Verification items for the finished model (mm, model axes). Round coordinates to 2 decimals unless told otherwise and drop trailing zeros. Loops run counter-clockwise (first coordinate to the right, second up) from the corner with the lowest first, then second, coordinate; pieces in that order, holes last.
Autodesk Inventor part; units mm, degrees
ref_plane "Work Plane1" through (37.5, 25, 0) normal (0, 1, 0) x (-1, 0, 0)
ref_plane "YZ Plane" through (0, 0, 0) normal (1, 0, 0) x (0, 1, 0)
ref_plane "XZ Plane" through (0, 0, 0) normal (0, 1, 0) x (-1, 0, 0)
ref_plane "Work Plane1" through (37.5, 25, 0) normal (0, 1, 0) x (-1, 0, 0)
sketch "Sketch1" plane through (37.5, 25, 0) normal (0, 1, 0) x (-1, 0, 0)
  line L0 (0, 0) -> (75, 0)
  line L1 (75, 0) -> (75, 100)
  line L2 (0, 100) -> (75, 100)
  line L3 (0, 0) -> (0, 100)
  circle A0 centre (6.75, 86) radius 2.7
  circle A1 centre (68.25, 86) radius 2.7
  circle A2 centre (68.25, 21.25) radius 2.7
  circle A3 centre (6.75, 21.25) radius 2.7
  line L4 (3, 3) -> (3, 17.5)
  line L5 (3, 17.5) -> (10.5, 17.5)
  line L6 (10.5, 17.5) -> (10.5, 25)
  line L7 (10.5, 25) -> (3, 25)
  line L8 (3, 25) -> (3, 77.25)
  arc A4 (8, 82.25) -> (3, 77.25) centre (8, 77.25) ccw
  line L9 (8, 82.25) -> (10.5, 82.25)
  line L10 (10.5, 82.25) -> (10.5, 89.75)
  line L11 (10.5, 89.75) -> (8, 89.75)
  arc A5 (3, 94.75) -> (8, 89.75) centre (8, 94.75) ccw
  line L12 (3, 94.75) -> (3, 97)
  line L13 (3, 97) -> (72, 97)
  line L14 (72, 97) -> (72, 94.75)
  arc A6 (67, 89.75) -> (72, 94.75) centre (67, 94.75) ccw
  line L15 (67, 89.75) -> (64.5, 89.75)
  line L16 (64.5, 89.75) -> (64.5, 82.25)
  line L17 (64.5, 82.25) -> (67, 82.25)
  arc A7 (72, 77.25) -> (67, 82.25) centre (67, 77.25) ccw
  line L18 (72, 77.25) -> (72, 25)
  line L19 (72, 25) -> (64.5, 25)
  line L20 (64.5, 25) -> (64.5, 17.5)
  line L21 (64.5, 17.5) -> (72, 17.5)
  line L22 (72, 17.5) -> (72, 3)
  line L23 (72, 3) -> (3, 3)
  line L24 (72, 55) -> (3, 55)
  point P0 (37.5, 0)
  dimension "d0" = 42
extrude "Extrusion1" add sketch "Sketch1" along normal blind 3 contours L3 L2 L1 L0 | L4 L5 L6 L7 L8 L24 L18 L19 L20 L21 L22 L23
properties part number "plytka"
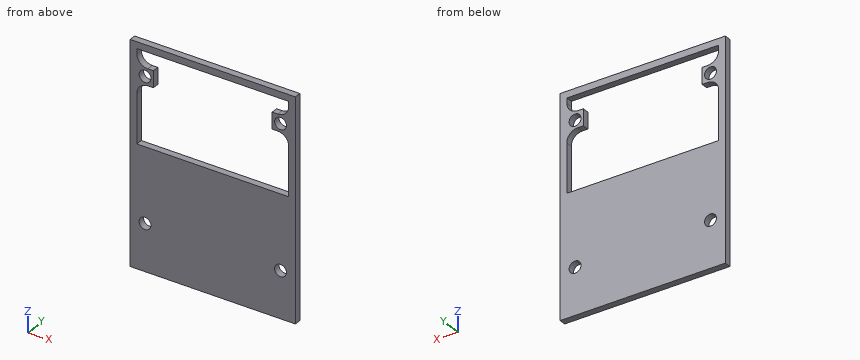
1. Section check C-C (z = 86). Enter the section's corners in (x, y).
2. Section check D-D (y = 27.45). Enter the section's corners in (x, z).
3. Section check B-B (x = 6). Enter the section's corners in (y, z), then the cut area to 3 significant figures.
4. Gauge pin test, flat end, axial feed: P1, Ø12, axis at x = -22, z = 64, coming from the -Y side. Record the tip position at first contact, or that the pin passes through.
5. Section check A-A (z = 21.25). Enter the section's corners in (x, y), then the cut area to 3 significant figures.
6. Scan lines: L1, parallel to X at y = 27, z = 67; L2, parallel to Z at x = -30.75, y = 26.1; L3, parallel to Z at x = 33.5, y = 25.6. Record each from-to range of solid material in increasing order.
Taken from the geometry:
1. outline: (-37.5, 25) - (-33.45, 25) - (-33.45, 28) - (-37.5, 28) - close; (-28.05, 25) - (-27, 25) - (-27, 28) - (-28.05, 28) - close; (27, 25) - (28.05, 25) - (28.05, 28) - (27, 28) - close; (33.45, 25) - (37.5, 25) - (37.5, 28) - (33.45, 28) - close
2. outline: (-37.5, 0) - (37.5, 0) - (37.5, 100) - (-37.5, 100) - close; hole (-34.5, 55) - (34.5, 55) - (34.5, 77.25) arc R5 ccw to (29.5, 82.25) - (27, 82.25) - (27, 89.75) - (29.5, 89.75) arc R5 ccw to (34.5, 94.75) - (34.5, 97) - (-34.5, 97) - (-34.5, 94.75) arc R5 ccw to (-29.5, 89.75) - (-27, 89.75) - (-27, 82.25) - (-29.5, 82.25) arc R5 ccw to (-34.5, 77.25) - close; hole circle Ø5.4 at (-30.75, 21.25); hole circle Ø5.4 at (-30.75, 86); hole circle Ø5.4 at (30.75, 21.25); hole circle Ø5.4 at (30.75, 86)
3. outline: (25, 0) - (28, 0) - (28, 55) - (25, 55) - close; (25, 97) - (28, 97) - (28, 100) - (25, 100) - close
3. area: 174 mm2
4. P1: passes through
5. outline: (-37.5, 25) - (-33.45, 25) - (-33.45, 28) - (-37.5, 28) - close; (-28.05, 25) - (28.05, 25) - (28.05, 28) - (-28.05, 28) - close; (33.45, 25) - (37.5, 25) - (37.5, 28) - (33.45, 28) - close
5. area: 193 mm2
6. L1: x = -37.5 to -34.5, 34.5 to 37.5
6. L2: z = 0 to 18.55, 23.95 to 55, 82.09 to 83.3, 88.7 to 89.91, 97 to 100
6. L3: z = 0 to 55, 80.25 to 91.75, 97 to 100
